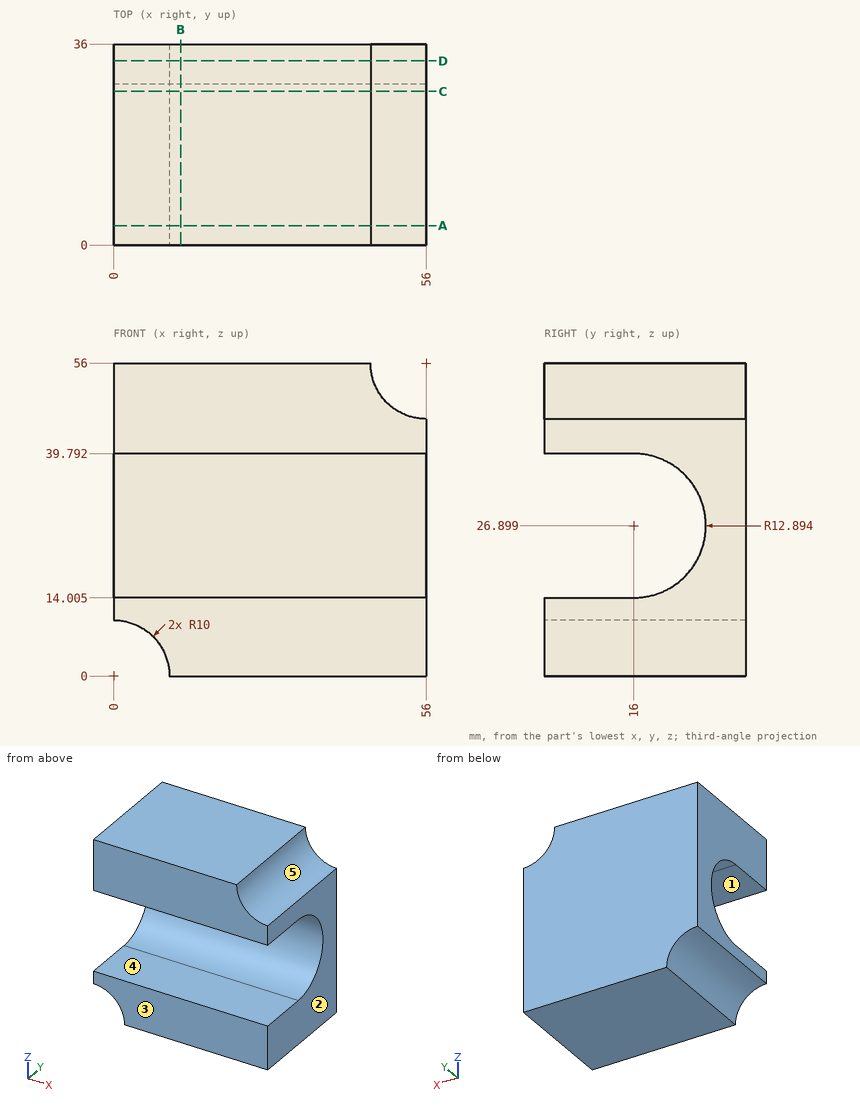
Answer from the drawing. Dimensions are ordinates in mm from the lowest x, y and z of the part. A direction names the side the tool comes from. Round coordinates to 2 decimals unless told otherwise and drop trailing zeros. Loops run counter-clockwise (first coordinate to the right, second up) from the corner with the lowest first, then second, coordinate; pieces in that order, holes last. Notation, with made-up numbers: M 10,76.5 L 52,76.5 A12 cw 52,90.5 Z; hole C 89,22.5 d7. An arc over 180 degrees is marked long. One line per question, with ' | ' between items. Start each with the question number.
(1) A cutting plane is placed at D-D on y = 33. Write down the section's boundary in (x, z).
(2) A cutting plane is placed at C-C on y = 27.5. Write down the section's boundary in (x, z), plus the area to 3 significant figures.
(3) A cutting plane is placed at A-A on y = 3.5. Write down the section's boundary in (x, z) (1 decimal), plus the area to 4 significant figures.
(4) For a pull along Z with two mould halves and no side action, classify the marked faces 3, 4 and 5 as released by +Z, released by -Z, zero draft, split by the parting line, or undercut.
(5) A tool of negligible diameter and unlimited length cuts with its end or side. For the marked faces 1 and 2, from which of +Z, -Z, +X, -X, +Y, -Y can it reach the whole face along a straight path? Write none if from no direction.
(6) A cutting plane is placed at B-B on x = 12. Write down the section's boundary in (y, z) (1 decimal).
(7) Find the intervals of material crossed by line 1 (Z direction, x = 37, y = 4) (1 decimal); line 2 (Y direction, x = 16.5, z = 26.5); line 3 (Z direction, x = 52, y = 22.5) (1 decimal), in increasing order.
(8) Flat-ended cylindrical pins translate along their axes: pin 1 Ø2 at (x, z) = (12, 33.5) entering from -Y (1 decimal); pin 2 Ø12 at (x, z) = (19.5, 27) entering from -Y; pin 3 Ø8 at (y, z) = (14, 19.5) entering from +X. Find the tip coordinate at first contact, or state that the pin passes through.
Geometry check:
1) outline: M 0,10 A10 cw 10,0 L 56,0 L 56,46 A10 cw 46,56 L 0,56 Z
2) outline: M 0,10 A10 cw 10,0 L 56,0 L 56,21.07 L 0,21.07 Z; M 0,32.73 L 56,32.73 L 56,46 A10 cw 46,56 L 0,56 Z | area: 2,330 mm²
3) outline: M 0,10 A10 cw 10,0 L 56,0 L 56,14 L 0,14 Z; M 0,39.8 L 56,39.8 L 56,46 A10 cw 46,56 L 0,56 Z | area: 1,535 mm²
4) face 3: zero draft | face 4: undercut | face 5: released by +Z
5) face 1: +X, -X, -Y | face 2: +Z, -Z, +X, +Y, -Y
6) outline: M 0,0 L 36,0 L 36,56 L 0,56 L 0,39.8 L 16,39.8 A12.9 cw 16,14 L 0,14 Z
7) line 1: z = 0 to 14, 39.8 to 56 | line 2: y = 28.89 to 36 | line 3: z = 0 to 15.8, 38 to 46.8
8) pin 1: stops at y = 26.4 | pin 2: stops at y = 27.36 | pin 3: passes through
